Read the model definition and answer for the solid it produces. Units are mm, in the model's axes. A direction names the side the tool comes from. Give positions to 0.01 mm unless a question says otherwise; leave off trailing zeros. Order: outer loops, then holes, each group sorted by start corner. A loop starts at its lowest first (then second) coordinate and runs counter-clockwise, first axis right, second up. Notation, with made-up numbers: (48, 7) - (107, 7) arc R26 ccw to (107, 22) - close; hole circle Ø9 at (70.25, -39). An arc over 180 degrees is marked (long way). Use a Markdown table: item, result. Add a question column.
1. Consider L1, parallel to Z at x = -30.5, y = 9; L2, parallel to Z at x = -14, y = 5; L3, parallel to Z at x = -17.5, y = 10.25. Determine where each line is inside the solid, lowest interval first.
2. A cutting plane is placed at D-D on x = -7. State how many separate pieces and enclosed holes the cut face has, and give its area (3 significant figures).
3. A cutting plane is placed at B-B on y = -3.75. Determine the outline of the cut face in (x, z), and give its area (3 significant figures).
4. For a pull along Y with two mould halves and no side action, classify faces 1 (the flat face through (-10.64, 2.85, -48.99)), 2 (the flat face through (-23, 8, -1)), 3 (the cylindrical face through (-11.145, 1.412, -48.009)), 4 (the flat face through (-26.144, 19.428, -0.493)) as released by +Y, released by -Y, zero draft, split by the parting line, or undercut.
5. Which of the six approach directions +Z, -Z, +X, -X, +Y, -Y give full straight-line access (tool end or side, diameter ignored) to faces 5 (the cylindrical face through (-39.28, 21.47, -0.49)), 6 (the flat face through (-29.77, 12.12, -48.9)), 7 (the flat face through (-22, 8, -97)), 8 (the flat face through (-26.403, 19.498, -97.493)), 9 (the flat face through (-11.251, 0.944, -12.173))?
6. Flat-ended cylindrical pins translate along their axes: P1, Ø4, axis at y = 3, z = -54, coming from the +X side; P2, Ø2, axis at y = 11.5, z = -39, coming from the +X side; P3, Ø6, axis at x = -32, y = -3.5, coming from the -Z side; P4, Ø3, axis at x = -30, z = -75, coming from the +Y side. Find the tip coordinate at first contact, or state that the pin passes through.
7. A cutting plane is placed at C-C on z = -37. Determine the outline of the cut face in (x, y).
8. A cutting plane is placed at A-A on z = -7.5. Determine the outline of the cut face in (x, y).
```python
from build123d import *

# Parameters (mm, degrees)
BOSS_EXTRUDE1_DEPTH = 1
BOSS_EXTRUDE2_DEPTH = 96
BOSS_EXTRUDE3_DEPTH = 1
BOSS_EXTRUDE4_DEPTH = 16
EXTRUDE_THIN1_REACH = 110.549
CUT_EXTRUDE1_DEPTH  = 102.965680501
CUT_EXTRUDE2_DEPTH  = 102.965680501
FILLET1_START       = -19
FILLET1_DEPTH       = 16
FILLET2_R           = 10
FILLET3_R           = 10
FILLET4_R           = 10
CHAMFER1_SIZE       = 1
CHAMFER2_SIZE       = 1
SKETCH8_R           = 1
CUT_EXTRUDE3_DEPTH  = 3


with BuildPart() as part:
    # Sketch1 → Boss-Extrude1 (new body)
    with BuildSketch(Plane.XY):
        with BuildLine():
            Line((-1.180699325, 1.221103194), (-15.635082302, 16.170119303))
            ThreePointArc((-15.635082302, 16.170119303), (-16.269985561, 16.670148445), (-17.01532588, 16.982556993))
            Line((-17.01532588, 16.982556993), (-35.53120451, 21.94387172))
            ThreePointArc((-35.53120451, 21.94387172), (-39.325299736, 21.444369607), (-41.654928867, 18.408337814))
            Line((-41.654928867, 18.408337814), (-44.243119318, 8.749079551))
            ThreePointArc((-44.243119318, 8.749079551), (-43.743617206, 4.954984325), (-40.707585412, 2.625355194))
            Line((-40.707585412, 2.625355194), (-4.96832984, -6.950949475))
            ThreePointArc((-4.96832984, -6.950949475), (-2.691872704, -6.651248207), (-1.294095226, -4.829629131))
            Line((-1.294095226, -4.829629131), (-0.43962256, -1.640693729))
            ThreePointArc((-0.43962256, -1.640693729), (-0.433194836, -0.11217799), (-1.180699325, 1.221103194))
        make_face()
    extrude(amount=-BOSS_EXTRUDE1_DEPTH)

    # Sketch2 → Boss-Extrude2 (add)
    with BuildSketch(Plane(origin=(0, 0, -1), x_dir=(-1, 0, 0), z_dir=(0, 0, -1))):
        Polygon((3.415415569, -1.155394517), (3.674234614, -2.121320344), (19.129047835, 2.019784378), (18.87022879, 2.985710204), align=None)
        Polygon((21.888124605, 11.041286214), (22.146943651, 10.075360388), (37.601756871, 14.216465109), (37.342937826, 15.182390936), align=None)
    extrude(amount=BOSS_EXTRUDE2_DEPTH)

    # Sketch3 → Boss-Extrude3 (add)
    with BuildSketch(Plane(origin=(0, 0, -97), x_dir=(-1, 0, 0), z_dir=(0, 0, -1))):
        with BuildLine():
            Line((4.96832984, -6.950949475), (40.707585412, 2.625355194))
            ThreePointArc((40.707585412, 2.625355194), (43.743617206, 4.954984325), (44.243119318, 8.749079551))
            Line((44.243119318, 8.749079551), (41.654928867, 18.408337814))
            ThreePointArc((41.654928867, 18.408337814), (39.325299736, 21.444369607), (35.53120451, 21.94387172))
            Line((35.53120451, 21.94387172), (17.01532588, 16.982556993))
            ThreePointArc((17.01532588, 16.982556993), (16.269985561, 16.670148445), (15.635082302, 16.170119303))
            Line((15.635082302, 16.170119303), (1.180699325, 1.221103194))
            ThreePointArc((1.180699325, 1.221103194), (0.433194836, -0.11217799), (0.43962256, -1.640693729))
            Line((0.43962256, -1.640693729), (1.294095226, -4.829629131))
            ThreePointArc((1.294095226, -4.829629131), (2.691872704, -6.651248207), (4.96832984, -6.950949475))
        make_face()
    extrude(amount=BOSS_EXTRUDE3_DEPTH)

    # Sketch4 → Boss-Extrude4 (add)
    with BuildSketch(Plane(origin=(-2.897777479, 0.776457135, 0), x_dir=(0, 0, -1), z_dir=(0.9659258262890703, -0.25881904510251386, 0))):
        with BuildLine():
            Line((49, 6), (49, -2))
            Line((49, -2), (65.5, -2))
            Line((65.5, -2), (65.5, 6))
            ThreePointArc((65.5, 6), (60.5, 1), (55.5, 6))
            Line((55.5, 6), (49, 6))
        make_face()
        with BuildLine():
            Line((32.5, 6), (32.5, -2))
            Line((32.5, -2), (49, -2))
            Line((49, -2), (49, 6))
            Line((49, 6), (42.5, 6))
            ThreePointArc((42.5, 6), (37.5, 1), (32.5, 6))
        make_face()
    extrude(amount=-BOSS_EXTRUDE4_DEPTH)

    # Extrude-Thin1: up to this face of the body (flat: up to its plane)
    extrude_thin1_end = Plane(part.part.faces().sort_by_distance((-42.949024093, 13.578708682, -97.5))[0])
    # Sketch5 → Extrude-Thin1 (add, up to the picked face)
    with BuildSketch(Plane(origin=(-2.897777479, 0.776457135, 0), x_dir=(0, 0, -1), z_dir=(0.9659258262890703, -0.25881904510251386, 0)), mode=Mode.PRIVATE) as extrude_thin1_sk1:
        with BuildLine():
            ThreePointArc((55.5, 6), (60.5, 1), (65.5, 6))
            ThreePointArc((65.5, 6), (60.5, 11), (55.5, 6))
        make_face()
        with BuildLine():
            ThreePointArc((56.5, 6), (60.5, 2), (64.5, 6))
            ThreePointArc((64.5, 6), (60.5, 10), (56.5, 6))
        make_face(mode=Mode.SUBTRACT)
    extrude_thin1_tool1 = split(extrude(extrude_thin1_sk1.sketch, amount=-EXTRUDE_THIN1_REACH, mode=Mode.PRIVATE), bisect_by=extrude_thin1_end, keep=Keep.BOTH, mode=Mode.PRIVATE)
    # Sketch5 → Extrude-Thin1 (add, up to the picked face)
    with BuildSketch(Plane(origin=(-2.897777479, 0.776457135, 0), x_dir=(0, 0, -1), z_dir=(0.9659258262890703, -0.25881904510251386, 0)), mode=Mode.PRIVATE) as extrude_thin1_sk2:
        with BuildLine():
            ThreePointArc((32.5, 6), (37.5, 1), (42.5, 6))
            ThreePointArc((42.5, 6), (37.5, 11), (32.5, 6))
        make_face()
        with BuildLine():
            ThreePointArc((33.5, 6), (37.5, 2), (41.5, 6))
            ThreePointArc((41.5, 6), (37.5, 10), (33.5, 6))
        make_face(mode=Mode.SUBTRACT)
    extrude_thin1_tool2 = split(extrude(extrude_thin1_sk2.sketch, amount=-EXTRUDE_THIN1_REACH, mode=Mode.PRIVATE), bisect_by=extrude_thin1_end, keep=Keep.BOTH, mode=Mode.PRIVATE)
    add(extrude_thin1_tool1.solids().sort_by(Axis((-2.602356, 1.878986, -60.5), (-0.9659258262890703, 0.25881904510251386, 0)))[0])
    add(extrude_thin1_tool2.solids().sort_by(Axis((-2.602356, 1.878986, -37.5), (-0.9659258262890703, 0.25881904510251386, 0)))[0])

    # Sketch6 → Cut-Extrude1 (cut, through all)
    with BuildSketch(Plane(origin=(-23.182219831, 6.211657082, 0), x_dir=(0, 0, -1), z_dir=(0.9659258262890705, -0.2588190451025127, 0))):
        with BuildLine():
            Line((57.035898385, 4), (63.964101615, 4))
            ThreePointArc((63.964101615, 4), (64.202459174, 4.486132084), (64.372983346, 5))
            Line((64.372983346, 5), (56.627016654, 5))
            ThreePointArc((56.627016654, 5), (56.797540826, 4.486132084), (57.035898385, 4))
        make_face()
    extrude(amount=-CUT_EXTRUDE1_DEPTH, mode=Mode.SUBTRACT)

    # Sketch7 → Cut-Extrude2 (cut, through all)
    with BuildSketch(Plane(origin=(-23.182219831, 6.211657082, 0), x_dir=(0, 0, -1), z_dir=(0.9659258262890704, -0.25881904510251263, 0))):
        with BuildLine():
            Line((34.035898385, 4), (40.964101615, 4))
            ThreePointArc((40.964101615, 4), (41.202459174, 4.486132084), (41.372983346, 5))
            Line((41.372983346, 5), (33.627016654, 5))
            ThreePointArc((33.627016654, 5), (33.797540826, 4.486132084), (34.035898385, 4))
        make_face()
    extrude(amount=-CUT_EXTRUDE2_DEPTH, mode=Mode.SUBTRACT)

    # Fillet1: read off the stored shape, not the designer's step
    # Fillet1 outline → Fillet1 (add)
    with BuildSketch(Plane(origin=(0, 0, 0), x_dir=(0.2588190451025141, 0.96592582628907, 0), z_dir=(0.9659258262890701, -0.2588190451025141, 0)).offset(FILLET1_START)):
        with BuildLine():
            ThreePointArc((6.666666667, -32.544643751), (0.472273473, -29.216737139), (-2, -22.633931253))
            Line((-2, -22.633931253), (-2, -32.5))
            Line((-2, -32.5), (6, -32.5))
            ThreePointArc((6, -32.5), (6.334079897, -32.511173422), (6.666666667, -32.544643751))
        make_face()
        with BuildLine():
            ThreePointArc((-2, -75.366068747), (0.472273473, -68.783262861), (6.666666667, -65.455356249))
            ThreePointArc((6.666666667, -65.455356249), (6.334079897, -65.488826578), (6, -65.5))
            Line((6, -65.5), (-2, -65.5))
            Line((-2, -65.5), (-2, -75.366068747))
        make_face()
    extrude(amount=FILLET1_DEPTH)

    # Fillet2
    # the kernel refuses this fillet: 10 mm, written as the material it adds along each edge
    with BuildSketch(Plane(origin=(-37.342937826, 15.182390936, -65.398979486), x_dir=(0, 0, -1), z_dir=(0.9659258262890703, -0.25881904510251386, 0))) as fillet2_piece_1:
        with BuildLine():
            CenterArc((7.101020514, 10), FILLET2_R, 216.869897646, 53.130102354)
            ThreePointArc((-0.898979486, 4), (-0.020664308, 2.096376317), (0, 0))
            Line((0, 0), (7.101020514, 0))
        make_face()
    extrude(amount=16)
    with BuildSketch(Plane(origin=(-37.342937826, 15.182390936, -32.601020514), x_dir=(0.25252017519049164, 0.9424181237471358, -0.21927526343546186), z_dir=(0.9659258262890703, -0.25881904510251386, 0))) as fillet2_piece_2:
        with BuildLine():
            CenterArc((8.199552211, 9.120955865), FILLET2_R, 192.666469307, 53.130102354)
            Line((-1.557078144, 6.92820323), (0, 0))
            ThreePointArc((0, 0), (2.049888053, 0.439522068), (4.099776106, 0))
        make_face()
    extrude(amount=16)

    # Fillet3
    # the kernel refuses this fillet: 10 mm, written as the material it adds along each edge
    with BuildSketch(Plane(origin=(-37.342937826, 15.182390936, -55.601020514), x_dir=(0.252520175190492, 0.9424181237471373, -0.21927526343545575), z_dir=(0.9659258262890703, -0.25881904510251386, 0))) as fillet3_piece_1:
        with BuildLine():
            CenterArc((8.199552211, 9.120955865), FILLET3_R, 192.666469307, 53.130102354)
            Line((-1.557078144, 6.92820323), (0, 0))
            ThreePointArc((0, 0), (2.049888053, 0.439522068), (4.099776106, 0))
        make_face()
    extrude(amount=16)
    with BuildSketch(Plane(origin=(-37.342937826, 15.182390936, -42.398979486), x_dir=(0, 0, -1), z_dir=(0.9659258262890703, -0.25881904510251386, 0))) as fillet3_piece_2:
        with BuildLine():
            CenterArc((7.101020514, 10), FILLET3_R, 216.869897646, 53.130102354)
            ThreePointArc((-0.898979486, 4), (-0.020664308, 2.096376317), (0, 0))
            Line((0, 0), (7.101020514, 0))
        make_face()
    extrude(amount=16)

    # Fillet4
    # the kernel refuses this fillet: 10 mm, written as the material it adds along each edge
    with BuildSketch(Plane(origin=(-1.344863208, 6.572012093, -42.5), x_dir=(0.24178159790789314, 0.9023412077274722, 0.35682208977308716), z_dir=(-0.9659258262890703, 0.25881904510251386, 0))) as fillet4_piece_1:
        with BuildLine():
            CenterArc((7.136441795, 9.34172359), FILLET4_R, 200.905157448, 48.189685104)
            Line((-2.205281794, 5.773502692), (-2.392116266, 5.702138274))
            Line((-2.392116266, 5.702138274), (-0.186834472, -0.071364418))
            Line((-0.186834472, -0.071364418), (0.071364418, -0.186834472))
            ThreePointArc((0.071364418, -0.186834472), (1.784110449, 0.129138205), (3.49685648, -0.186834472))
            Line((3.49685648, -0.186834472), (3.568220898, 0))
        make_face()
    extrude(amount=16)
    with BuildSketch(Plane(origin=(-1.344863208, 6.572012093, -55.5), x_dir=(0.24178159790789344, 0.9023412077274733, -0.3568220897730836), z_dir=(-0.9659258262890703, 0.25881904510251386, 0))) as fillet4_piece_2:
        with BuildLine():
            CenterArc((7.136441795, -9.34172359), FILLET4_R, 110.905157448, 48.189685104)
            Line((-2.205281794, -5.773502692), (-2.392116266, -5.702138274))
            Line((-2.392116266, -5.702138274), (-0.186834472, 0.071364418))
            Line((-0.186834472, 0.071364418), (0.071364418, 0.186834472))
            ThreePointArc((0.071364418, 0.186834472), (1.784110449, -0.129138205), (3.49685648, 0.186834472))
            Line((3.49685648, 0.186834472), (3.568220898, 0))
        make_face()
    extrude(amount=16)

    # Chamfer1
    chamfer1_edges = [part.edges().sort_by_distance(p)[0] for p in [
        (-11.142822179, 0.915157844, -1),
        (-11.142822179, 0.915157844, -97),
    ]]
    chamfer(chamfer1_edges, length=CHAMFER1_SIZE)

    # Chamfer2
    chamfer2_edges = [part.edges().sort_by_distance(p)[0] for p in [
        (-29.615531216, 13.111838575, -1),
        (-29.615531216, 13.111838575, -97),
    ]]
    chamfer(chamfer2_edges, length=CHAMFER2_SIZE)

    # Sketch8 → Cut-Extrude3 (cut)
    with BuildSketch(Plane(origin=(-0.776457135, -2.897777479, 0), x_dir=(0.9659258262890701, -0.25881904510251413, 0), z_dir=(-0.25881904510251413, -0.9659258262890701, 0))):
        with Locations((-11, -49)):
            Circle(SKETCH8_R)
    extrude(amount=-CUT_EXTRUDE3_DEPTH, mode=Mode.SUBTRACT)


solid = part.part
```
Output values:
| question | item | result |
|---|---|---|
| 1 | L1 | -98 to -97, -1 to 0 |
| 1 | L2 | -98 to -97, -68.03 to -29.97, -1 to 0 |
| 1 | L3 | -98 to -97, -65.46 to -64.45, -56.55 to -55.54, -42.46 to -41.45, -33.55 to -32.54, -1 to 0 |
| 2 | separate pieces | 1 |
| 2 | enclosed holes | 2 |
| 2 | area | 430 mm² |
| 3 | outline | (-16.91, -98) - (-1, -98) - (-1, -97) - (-16.91, -97) - close; (-16.91, -1) - (-1, -1) - (-1, 0) - (-16.91, 0) - close |
| 3 | area | 31.8 mm² |
| 4 | face 1 | undercut |
| 4 | face 2 | zero draft |
| 4 | face 3 | undercut |
| 4 | face 4 | released by +Y |
| 5 | face 5 | +Z, +Y |
| 5 | face 6 | -X, -Y |
| 5 | face 7 | none |
| 5 | face 8 | +Z, -Z, +X, +Y |
| 5 | face 9 | +X, +Y |
| 6 | P1 | x = -1.77 |
| 6 | P2 | x = -0.06 |
| 6 | P3 | through |
| 6 | P4 | y = 13.62 |
| 7 | outline | (-43.2, 12.64) - (-18.09, 5.91) - (-19.13, 2.02) - (-3.67, -2.12) - (-2.37, 2.74) - (-42.94, 13.61) - close; (-40.89, 21.28) - (-0.32, 10.41) - (-0.06, 11.38) - (-40.63, 22.25) - close |
| 8 | outline | (-37.6, 14.22) - (-22.15, 10.08) - (-21.89, 11.04) - (-37.34, 15.18) - close; (-19.13, 2.02) - (-3.67, -2.12) - (-3.42, -1.16) - (-18.87, 2.99) - close |
